Verification items for the finished model (mm, model axes). Round coordinates to 2 decimals unless told otherwise and drop trailing zeros. Loops run counter-clockwise (first coordinate to the right, second up) from the corner with the lowest first, then second, coordinate; pieces in that order, holes last. Notation, with made-up numbers: (-27.75, 7) - (8.25, 7) arc R26 cw to (8.25, 42) - close; hole circle Ø9 at (85.25, 11.5). An arc over 180 degrees is marked (long way). Use a Markdown table: item, result. Add a question column.
```python
from build123d import *

# Parameters (mm, degrees)
SKETCH1_R           = 1.5
BOSS_EXTRUDE1_DEPTH = 1
SKETCH2_R           = 1
BOSS_EXTRUDE2_DEPTH = 6
CUT_EXTRUDE1_DEPTH  = 0.75
FILLET1_R           = 0.5


with BuildPart() as part:
    # Sketch1 → Boss-Extrude1 (new body)
    with BuildSketch(Plane.XY):
        Circle(SKETCH1_R)
    extrude(amount=BOSS_EXTRUDE1_DEPTH)

    # Sketch2 → Boss-Extrude2 (add)
    with BuildSketch(Plane.XY.offset(1)):
        Circle(SKETCH2_R)
    extrude(amount=BOSS_EXTRUDE2_DEPTH)

    # Sketch3 → Cut-Extrude1 (cut)
    with BuildSketch(Plane(origin=(0, 0, 0), x_dir=(-1, 0, 0), z_dir=(0, 0, -1))):
        Polygon((0.261487369, -0.51474041), (0.576521955, -0.030915501), (0.315034587, 0.483824909), (-0.261487369, 0.51474041), (-0.576521955, 0.030915501), (-0.315034587, -0.483824909), align=None)
    extrude(amount=-CUT_EXTRUDE1_DEPTH, mode=Mode.SUBTRACT)

    # Fillet1
    fillet1_edges = [part.edges().sort_by_distance(p)[0] for p in [
        (-1.5, 0, 0),
    ]]
    fillet(fillet1_edges, radius=FILLET1_R)


solid = part.part
```
Q1. Section check B-B on z = 4.25. Record the cut outline in (x, y).
Q2. Go/stop test with flat-tipped pins: pin 1 Ø0.5 at (x, y) = (0, 0) entering from -Z; pin 2 Ø1.5 at (y, z) = (-0.5, 2.5) entering from -X. Record where each tip stops, or that it passes through.
Q3. Section check A-A on x = 0. Record the cut outline in (y, z).
Q4. Thickness scan on line 1 along Z through (x, y) = (0.5, -0.05); line 2 along Y through (x, z) = (0, 1.5). Record the ranges inside material, lowest first.
Q5. Release check for a two-part mould opening along Y. For faces 1 (the face through (0, 0, 0.75)), 2 (the face through (0, -1, 4)), 3 (the face through (0, -0.7, 0)) record: +Y half, -Y half, draft (parallel to the pull), parting line (faces both ways), or undercut.
Determined:
| question | item | result |
|---|---|---|
| 1 | outline | circle Ø2 at (0, 0) |
| 2 | pin 1 | stops at z = 0.75 |
| 2 | pin 2 | stops at x = -1 |
| 3 | outline | (-1.5, 0.5) arc R0.5 ccw to (-1, 0) - (-0.5, 0) - (-0.5, 0.75) - (0.5, 0.75) - (0.5, 0) - (1, 0) arc R0.5 ccw to (1.5, 0.5) - (1.5, 1) - (1, 1) - (1, 7) - (-1, 7) - (-1, 1) - (-1.5, 1) - close |
| 4 | line 1 | z = 0.75 to 7 |
| 4 | line 2 | y = -1 to 1 |
| 5 | face 1 | undercut |
| 5 | face 2 | parting line |
| 5 | face 3 | draft |
